CAD build for the part. Positions are in the model's coordinates, mm. Face numbers are marked on the shaded views. A direction names the side the tool comes from. Give positions to 0.01 mm unless a question says otherwise; leave off trailing zeros. Write each loop counter-clockwise with the first axis right and the second up, starting at its lowest first coordinate (ties: lowest second). Pieces come first, ordered by that corner, then holes. Notation, with made-up numbers: (31, -35.75) -> (86, -35.75) arc R31 ccw to (86, 1.25) -> close; hole circle Ø5 at (-3.75, 38.25). An arc over 180 degrees is marked (long way). Answer as a JSON object with one key per item and string values.
Autodesk Inventor part; units mm, degrees
ref_plane "YZ Plane" through (0, 0, 0) normal (1, 0, 0) x (0, 1, 0)
ref_plane "XZ Plane" through (0, 0, 0) normal (0, 1, 0) x (-1, 0, 0)
ref_plane "XY Plane" through (0, 0, 0) normal (0, 0, 1) x (1, 0, 0)
sketch "Sketch1" plane through (0, 0, 0) normal (0, 1, 0) x (-1, 0, 0)
  line L0 (0, 0) -> (-20.32, 0)
  line L1 (-20.32, 0) -> (-20.32, -76.2)
  line L2 (-20.32, -76.2) -> (0, -76.2)
  line L3 (0, -76.2) -> (0, 0)
  dimension "d0" = 20.32
  dimension "d1" = 76.2
extrude "Extrusion1" add sketch "Sketch1" along normal blind 7.62
sketch "Sketch2" plane through (0, 7.62, 0) normal (0, 1, 0) x (1, 0, 0)
  line L0 (0, 76.2) -> (0, 0)
  line L1 (0, 0) -> (0, 12.7)
  line L2 (0, 12.7) -> (20.32, 12.7)
  line L3 (20.32, 12.7) -> (20.32, 63.5)
  line L4 (20.32, 63.5) -> (0, 63.5)
  line L5 (0, 63.5) -> (0, 12.7)
  dimension "d4" = 12.7
  dimension "d5" = 20.32
  dimension "d6" = 50.8
extrude "Extrusion2" add sketch "Sketch2" along normal blind 43.18
sketch "Sketch3" plane through (20.32, 0, 0) normal (1, 0, 0) x (0, 0, -1)
  line L0 (12.7, 50.8) -> (63.5, 50.8)
  line L1 (38.1, 50.8) -> (38.1, 25.4)
  circle A0 centre (38.1, 25.4) radius 19.177
  point P0 (0, 0)
  dimension "d9" = 25.4
  dimension "d10" = 38.354
extrude "Extrusion3" cut sketch "Sketch3" against normal blind 43.18
fillet "Fillet1" radius 25.4 2 edges at (10.16, 50.8, -12.7) (10.16, 50.8, -63.5)
sketch "Sketch4" plane through (0, 7.62, 0) normal (0, 1, 0) x (1, 0, 0)
  line L0 (0, 0) -> (20.32, 0)
  line L1 (10.16, 0) -> (10.16, 6.35)
  line L2 (20.32, 76.2) -> (0, 76.2)
  line L3 (10.16, 76.2) -> (10.16, 69.85)
  dimension "d14" = 6.35
  dimension "d15" = 6.35
fillet "Fillet2" radius 25.4 1 edges at (10.16, 7.62, -12.7)
fillet "Fillet3" radius 25.4 1 edges at (10.16, 7.62, -63.5)
hole "Hole1" at (10.16, 7.62, -6.35) at (10.16, 7.62, -69.85) direction (0, -1, 0) diameter 5.08 end through all counterbore diameter 10.16 counterbore depth 3.81
sketch "Sketch5" plane through (10.16, 7.62, -6.35) normal (0, -1, 0) x (1, 0, 0)
  circle A0 centre (0, 0) radius 5.08
  circle A1 centre (0, -63.5) radius 2.54
  line L0 (-2.54, -63.5) -> (0, -63.5)
  circle A2 centre (0, -63.5) radius 5.08
  point P0 (-10.16, 6.35)
  dimension "d25" = 10.16
  dimension "d26" = 10.16
extrude "Extrusion4" cut sketch "Sketch5" against normal blind 43.18 contours A0 | A1 | A2
properties part number "Motor Mount Back Side"
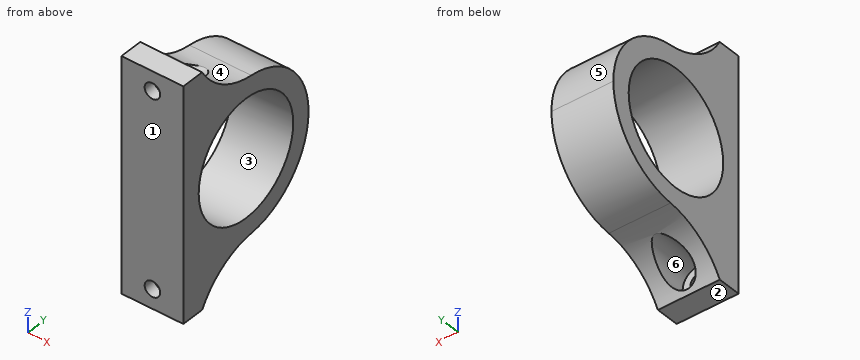
1) Mould opens along Y. For the marked faces 1, 2, 3 and 4 say: released by +Y, released by -Y, zero draft, split by the parting line, or undercut.
Model answer:
{"face 1": "released by -Y", "face 2": "zero draft", "face 3": "undercut", "face 4": "released by +Y"}
2) Slice it at D-D (y = 25.4). List the corners of the cut face in (x, z), then the cut area to 3 significant figures.
Model answer:
{"outline": "(0, -63.69) -> (20.32, -63.69) -> (20.32, -57.28) -> (0, -57.28) -> close; (0, -18.92) -> (20.32, -18.92) -> (20.32, -12.51) -> (0, -12.51) -> close", "area": "260 mm2"}
3) Slice it at B-B (y = 38.5). List the corners of the cut face in (x, z).
Model answer:
{"outline": "(0, -59.86) -> (20.32, -59.86) -> (20.32, -52.11) -> (0, -52.11) -> close; (0, -24.09) -> (20.32, -24.09) -> (20.32, -16.34) -> (0, -16.34) -> close"}
4) 3-axis set-ups, long thin cutter, end or side, ignore diameter. For the marked faces 5 and 6: which of +Z, -Z, +X, -X, +Y, -Y reach the whole face in a straight line?
Model answer:
{"face 5": "+Z, +X, -X, +Y", "face 6": "+Y"}
5) Slice it at A-A (z = -71). List the corners of the cut face in (x, y).
Model answer:
{"outline": "(0, 0) -> (7.9, 0) -> (7.9, 3.81) -> (5.21, 3.81) -> (5.21, 11.52) -> (0, 11.52) -> close; (12.42, 0) -> (20.32, 0) -> (20.32, 11.52) -> (15.11, 11.52) -> (15.11, 3.81) -> (12.42, 3.81) -> close"}
6) Pin check, flat tips, straight feed: pin 1 (8 mm diameter, centred on x = 8, z = -4.5, fed in from +Y); pin 2 (1 mm diameter, centred on y = 5.5, z = -15, fed in from -X); pin 3 (10 mm diameter, centred on x = 15.5, z = -63.5, fed in from +Y); pin 4 (2 mm diameter, centred on x = 14.5, y = 10.5, fed in from +Z). Stop position of each tip, or through.
Model answer:
{"pin 1": "stops at y = 13.87", "pin 2": "stops at x = 0", "pin 3": "stops at y = 40.53", "pin 4": "stops at z = -2.85"}
7) Wall check: probe 1 along Z at (x, y) = (10.16, 1.5); probe 2 along Z at (x, y) = (8.5, 3); probe 3 along Y at (x, z) = (17, -31). Give the ranges that are in metal, low to high.
Model answer:
{"probe 1": "z = -76.2 to -72.39, -67.31 to -8.89, -3.81 to 0", "probe 2": "z = -76.2 to -71.77, -67.93 to -8.27, -4.43 to 0", "probe 3": "y = 0 to 7.59, 43.21 to 49.79"}
8) Slice it at C-C (z = -6.35). List the corners of the cut face in (x, y).
Model answer:
{"outline": "(0, 0) -> (7.62, 0) -> (7.62, 3.81) -> (5.08, 3.81) -> (5.08, 12.72) -> (0, 12.72) -> close; (12.7, 0) -> (20.32, 0) -> (20.32, 12.72) -> (15.24, 12.72) -> (15.24, 3.81) -> (12.7, 3.81) -> close"}
